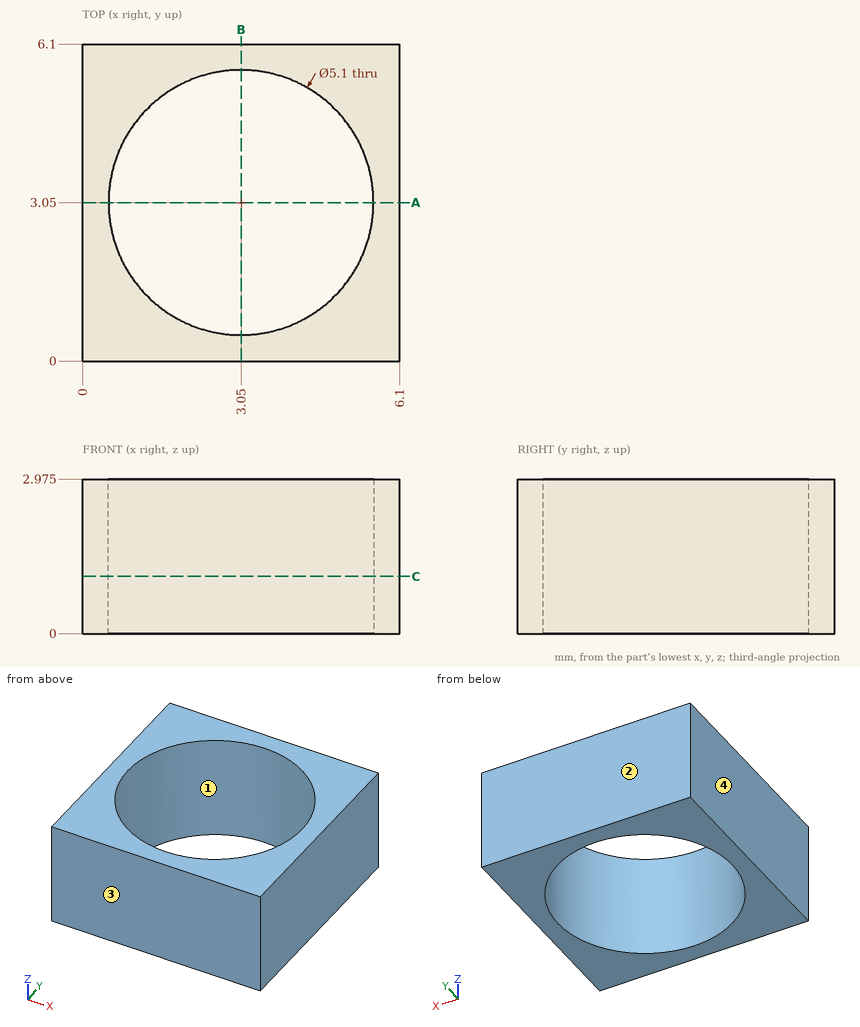
Could you check a few things on this drawing? It's one solid part, dimensions in mm from its lowest x, y, z. Coordinates: 2 decimals unless noted, no trailing zeros. Loops run counter-clockwise (first coordinate to the right, second up) from the corner with the lowest first, then second, coordinate; pieces in that order, holes last.
1. Imagine slicing it at A-A (y = 3.05). Please give me the cut outline in (x, z) (3 decimals), and give its area (4 significant figures).
2. We'd pull the mould along Y, two halves only. Please class the marked faces 1, 2, 3 and 4: released by +Y, released by -Y, zero draft, split by the parting line, or undercut.
3. I need wall thicknesses on L1, parallel to Y at x = 3, z = 2.8; L2, parallel to Y at x = 4, z = 0.9; L3, parallel to X at y = 0.75, z = 1.75. Which ranges of each line are inside material? Lowest first, please.
4. Imagine slicing it at C-C (z = 1.1). Please give me the cut outline in (x, y), and give its area (3 significant figures).
5. For P1, Ø3, axis at x = 3.05, y = 3.05, coming from the -Z side, with a flat end and sliding along its axis, tell me the tip position at first contact or that it passes through.
Computed values:
1. outline: (0, 0) - (0.5, 0) - (0.5, 2.975) - (0, 2.975) - close; (5.6, 0) - (6.1, 0) - (6.1, 2.975) - (5.6, 2.975) - close
1. area: 2.975 mm2
2. face 1: undercut
2. face 2: released by +Y
2. face 3: released by -Y
2. face 4: zero draft
3. L1: y = 0 to 0.5, 5.6 to 6.1
3. L2: y = 0 to 0.68, 5.42 to 6.1
3. L3: x = 0 to 1.95, 4.15 to 6.1
4. outline: (0, 0) - (6.1, 0) - (6.1, 6.1) - (0, 6.1) - close; hole circle Ø5.1 at (3.05, 3.05)
4. area: 16.8 mm2
5. P1: passes through
